Read the model definition and answer for the solid it produces. Units are mm, in the model's axes. Give positions to 0.01 mm unless a question says otherwise; leave off trailing zeros. Write each loop counter-clockwise with the first axis right and the second up, starting at its lowest first coordinate (ties: lowest second). Pieces come first, ordered by that corner, then holes. Notation, with made-up numbers: (37.5, -21.5) -> (50.5, -21.5) arc R13 cw to (50.5, -6.5) -> close; hole circle Ø2 at (46.25, 69.5). An arc over 180 degrees is marked (long way). Write item = value, one per line.
from build123d import *

# Parameters (mm, degrees)
SKETCH1_W           = 16
SKETCH1_H           = 4.5
BOSS_EXTRUDE1_DEPTH = 50
FILLET1_R           = 1.5
SKETCH2_R           = 2.5
CUT_EXTRUDE1_DEPTH  = 5


with BuildPart() as part:
    # Sketch1 → Boss-Extrude1 (new body)
    with BuildSketch(Plane.XY):
        Rectangle(SKETCH1_W, SKETCH1_H)
    extrude(amount=BOSS_EXTRUDE1_DEPTH)

    # Fillet1
    fillet1_edges = [part.edges().sort_by_distance(p)[0] for p in [
        (-8, 0, 50),
        (0, -2.25, 50),
        (8, 0, 50),
        (0, -2.25, 0),
        (-8, 0, 0),
        (0, 2.25, 0),
        (8, 0, 0),
        (0, 2.25, 50),
        (8, -2.25, 25),
        (-8, -2.25, 25),
        (-8, 2.25, 25),
        (8, 2.25, 25),
    ]]
    fillet(fillet1_edges, radius=FILLET1_R)

    # Sketch2 → Cut-Extrude1 (cut)
    with BuildSketch(Plane.XZ.offset(2.25)):
        with Locations(Location((0, 15, 0), (0, 0, 270))):
            Circle(SKETCH2_R)
        with Locations(Location((0, 35, 0), (0, 0, 270))):
            Circle(SKETCH2_R)
    extrude(amount=-CUT_EXTRUDE1_DEPTH, mode=Mode.SUBTRACT)


solid = part.part
(1) The part is cut by section A-A on z = 35. Determine the outline of the cut face in (x, y), plus the area to 3 significant figures.
Checks:
outline = (-8, -0.75) arc R1.5 ccw to (-6.5, -2.25) -> (-2.5, -2.25) -> (-2.5, 2.25) -> (-6.5, 2.25) arc R1.5 ccw to (-8, 0.75) -> close; (2.5, -2.25) -> (6.5, -2.25) arc R1.5 ccw to (8, -0.75) -> (8, 0.75) arc R1.5 ccw to (6.5, 2.25) -> (2.5, 2.25) -> close
area = 47.6 mm²
(2) Consider L1, parallel to Z at x = 2, y = -1.85; L2, parallel to X at y = -0.85, z = 32; L3, parallel to X at y = 0.1, z = 15. Determine where each line is inside the solid, lowest interval first.
Checks:
L1 = 0.48 to 13.5, 16.5 to 33.5, 36.5 to 49.52
L2 = -8 to 8
L3 = -8 to -2.5, 2.5 to 8
(3) The part is cut by section D-D on z = 19. Determine the outline of the cut face in (x, y).
Checks:
outline = (-8, -0.75) arc R1.5 ccw to (-6.5, -2.25) -> (6.5, -2.25) arc R1.5 ccw to (8, -0.75) -> (8, 0.75) arc R1.5 ccw to (6.5, 2.25) -> (-6.5, 2.25) arc R1.5 ccw to (-8, 0.75) -> close
(4) Given P1, Ø4.5, axis at x = 0, z = 35, coming from the -Y side, flat-ended and moving along its own axis, determine where the tip first touches the part or whether it passes through.
Checks:
P1 = through
(5) The part is cut by section C-C on y = -1.7. Determine the outline of the cut face in (x, z), plus the area to 3 significant figures.
Checks:
outline = (-7.66, 1.5) arc R1.16 ccw to (-6.5, 0.34) -> (6.5, 0.34) arc R1.16 ccw to (7.66, 1.5) -> (7.66, 48.5) arc R1.16 ccw to (6.5, 49.66) -> (-6.5, 49.66) arc R1.16 ccw to (-7.66, 48.5) -> close; hole circle Ø5 at (0, 15); hole circle Ø5 at (0, 35)
area = 715 mm²
(6) For a pull along Z with two mould halves and no side action, classify faces 1 (the cylindrical face through (7.57, 0.01, 49.55)), 2 (the cylindrical face through (0.1, 0, 17.5)), 3 (the cylindrical face through (7.57, 1.8, 25.33)), 4 (the cylindrical face through (-0.96, -0.03, 32.69)) as released by +Z, released by -Z, zero draft, split by the parting line, or undercut.
Checks:
face_1 = released by +Z
face_2 = undercut
face_3 = zero draft
face_4 = undercut
(7) The part is cut by section B-B on x = 0. Determine the outline of the cut face in (y, z), plus the area to 3 significant figures.
Checks:
outline = (-2.25, 1.5) arc R1.5 ccw to (-0.75, 0) -> (0.75, 0) arc R1.5 ccw to (2.25, 1.5) -> (2.25, 12.5) -> (-2.25, 12.5) -> close; (-2.25, 17.5) -> (2.25, 17.5) -> (2.25, 32.5) -> (-2.25, 32.5) -> close; (-2.25, 37.5) -> (2.25, 37.5) -> (2.25, 48.5) arc R1.5 ccw to (0.75, 50) -> (-0.75, 50) arc R1.5 ccw to (-2.25, 48.5) -> close
area = 178 mm²
